```python
from build123d import *

# Parameters (mm, degrees)
ESQUISSE1_R             = 37.5
BOSS_EXTRU_1_DEPTH      = 1.5
ESQUISSE2_R             = 17.5
BOSS_EXTRU_2_DEPTH      = 8
ESQUISSE4_W             = 20
ESQUISSE4_H             = 72.283474197
BOSS_EXTRU_5_DEPTH      = 25
ESQUISSE11_W            = 52.283474197
ESQUISSE11_H            = 25
ENL_V_MAT_EXTRU_5_DEPTH = 25
ESQUISSE12_R            = 3.5
ENL_V_MAT_EXTRU_8_DEPTH = 87.749161989
ESQUISSE13_W            = 5
ESQUISSE13_H            = 30
ENL_V_MAT_EXTRU_9_DEPTH = 12


with BuildPart() as part:
    # Esquisse1 → Boss.-Extru.1 (new body)
    with BuildSketch(Plane(origin=(0, 0, 0), x_dir=(1, 0, 0), z_dir=(0, 1, 0))):
        with Locations(Location((0, 0, 0), (0, 0, 270))):
            Circle(ESQUISSE1_R)
    extrude(amount=BOSS_EXTRU_1_DEPTH)

    # Esquisse2 → Boss.-Extru.2 (add)
    with BuildSketch(Plane(origin=(0, 1.5, 0), x_dir=(1, 0, 0), z_dir=(0, 1, 0))):
        with Locations(Location((0, 0, 0), (0, 0, 270))):
            Circle(ESQUISSE2_R)
    extrude(amount=-BOSS_EXTRU_2_DEPTH)

    # Esquisse4 → Boss.-Extru.5 (add)
    with BuildSketch(Plane(origin=(0, 1.5, 0), x_dir=(1, 0, 0), z_dir=(0, 1, 0))):
        with Locations((-0.151898301, -0.042028501)):
            Rectangle(ESQUISSE4_W, ESQUISSE4_H)
    extrude(amount=BOSS_EXTRU_5_DEPTH)

    # Esquisse11 → Enlèv. mat.-Extru.5 (cut)
    with BuildSketch(Plane(origin=(9.848101699, 0, 0), x_dir=(0, 0, -1), z_dir=(1, 0, 0))):
        with Locations((-0.0420285, 14)):
            Rectangle(ESQUISSE11_W, ESQUISSE11_H)
    extrude(amount=-ENL_V_MAT_EXTRU_5_DEPTH, mode=Mode.SUBTRACT)

    # Esquisse12 → Enlèv. mat.-Extru.8 (cut, through all)
    with BuildSketch(Plane(origin=(0, 0, -36.099708598), x_dir=(-1, 0, 0), z_dir=(0, 0, -1))):
        with Locations((0.151898301, 18.5)):
            Circle(ESQUISSE12_R)
    extrude(amount=-ENL_V_MAT_EXTRU_8_DEPTH, mode=Mode.SUBTRACT)

    # Esquisse13 → Enlèv. mat.-Extru.9 (cut)
    with BuildSketch(Plane(origin=(0, 1.5, 0), x_dir=(1, 0, 0), z_dir=(0, 1, 0))):
        Rectangle(ESQUISSE13_W, ESQUISSE13_H)
    extrude(amount=-ENL_V_MAT_EXTRU_9_DEPTH, mode=Mode.SUBTRACT)


solid = part.part
```
Here's how the part is built. I have some questions about the finished solid (model axes, mm). A direction names the side the tool comes from. Round coordinates to 2 decimals unless told otherwise and drop trailing zeros. Loops run counter-clockwise (first coordinate to the right, second up) from the corner with the lowest first, then second, coordinate; pieces in that order, holes last.
1. Suppose I cut it at B-B, the plane z = 0. Please give me the cut outline in (x, y), and give its area (3 significant figures).
Answers:
outline: (-37.5, 0) - (-17.5, 0) - (-17.5, -6.5) - (-2.5, -6.5) - (-2.5, 1.5) - (-37.5, 1.5) - close; (2.5, -6.5) - (17.5, -6.5) - (17.5, 0) - (37.5, 0) - (37.5, 1.5) - (2.5, 1.5) - close
area: 300 mm2
2. Suppose I cut it at D-D, the plane z = -27.5. Please give me the cut outline in (x, y).
Answers:
outline: (-25.5, 0) - (25.5, 0) - (25.5, 1.5) - (9.85, 1.5) - (9.85, 26.5) - (-10.15, 26.5) - (-10.15, 1.5) - (-25.5, 1.5) - close; hole circle Ø7 at (-0.15, 18.5)
3. Suppose I cut it at C-C, the plane y = 24.5. Please give me the cut outline in (x, z), and give its area (3 significant figures).
Answers:
outline: (-10.15, -36.1) - (9.85, -36.1) - (9.85, -26.1) - (-10.15, -26.1) - close; (-10.15, 26.18) - (9.85, 26.18) - (9.85, 36.18) - (-10.15, 36.18) - close
area: 400 mm2
4. For faces 1 (the face through (0, 14, -26.1)), 2 (the face through (-10.152, 14, 31)), 3 (the face through (0, -2, 15)), 4 (the face through (9.848, 14, -31)), 5 (the face through (0, 14, -36.1)), which set-ups out of +Z, -Z, +X, -X, +Y, -Y let a thin tool reach every point of the face, with its end or its side?
Answers:
face 1: +X, -X, +Y
face 2: +Z, -Z, -X, +Y
face 3: +Y, -Y
face 4: +Z, -Z, +X, +Y
face 5: -Z, +X, -X, +Y
5. Thinking about a two-plate mould opening in Z: for faces 6 (the face through (0, -2, -15)), 7 (the face through (0, 14, 26.184)), 8 (the face through (-10.648, -3.204, -13.887)), 9 (the face through (0.3, 21.97, 31.11)), which applies, released by +Z, released by -Z, zero draft, split by the parting line, or undercut?
Answers:
face 6: undercut
face 7: undercut
face 8: split by the parting line
face 9: zero draft
6. Suppose I cut it at A-A, the plane y = 18.5. Please give me the cut outline in (x, z), and give its area (3 significant figures).
Answers:
outline: (-10.15, -36.1) - (-3.65, -36.1) - (-3.65, -26.1) - (-10.15, -26.1) - close; (-10.15, 26.18) - (-3.65, 26.18) - (-3.65, 36.18) - (-10.15, 36.18) - close; (3.35, -36.1) - (9.85, -36.1) - (9.85, -26.1) - (3.35, -26.1) - close; (3.35, 26.18) - (9.85, 26.18) - (9.85, 36.18) - (3.35, 36.18) - close
area: 260 mm2
7. Will these pins go through, and if not, where does the flat tip stop? pin 1 (2.5 mm diameter, centred on y = -4.5, z = 3.5, fed in from +X); pin 2 (5 mm diameter, centred on y = 16, z = 29.5, fed in from -X); pin 3 (16 mm diameter, centred on x = -0.5, y = 18, fed in from -Z); pin 4 (1.5 mm diameter, centred on x = -1, z = -10.5, fed in from -Y).
Answers:
pin 1: stops at x = 17.35
pin 2: stops at x = -10.15
pin 3: stops at z = -36.1
pin 4: passes through
8. If I drill on probe 1 along Z at (x, y) = (1, 1); probe 2 along Z at (x, y) = (0.5, 5); probe 3 along Y at (x, z) = (-34, 1.5), over which ranges is the centre line in solid material (lowest first)?
Answers:
probe 1: z = -37.49 to -15, 15 to 37.49
probe 2: z = -36.1 to -26.1, 26.18 to 36.18
probe 3: y = 0 to 1.5
